Read the model definition and answer for the solid it produces. Units are mm, in the model's axes. A direction names the side the tool comes from. Coordinates: 2 decimals unless noted, no trailing zeros. Write each loop counter-clockwise with the first axis right and the second up, starting at its lowest first coordinate (ties: lowest second). Pieces come first, ordered by that corner, then holes. Notation, with made-up numbers: (31, 17) - (35, 17) arc R34 cw to (35, 55) - close; hole circle Ø4 at (87, 8). An arc over 180 degrees is marked (long way). Return JSON: item names as keys, results as strings.
```python
from build123d import *

# Parameters (mm, degrees)
F0_R     = 24
F0_R_2   = 19
F1_DEPTH = 60
F2_R     = 24
F2_R_2   = 19
F3_DEPTH = 10
F4_R     = 24
F4_R_2   = 19
F5_DEPTH = 10
F6_R     = 9
F7_DEPTH = 25


with BuildPart() as f1:
    # F0 (on Front) → F1 (new body, symmetric)
    with BuildSketch(Plane.XZ):
        with BuildLine():
            Line((83, 13.3241766691), (83, 33.3241766691))
            Line((83, 33.3241766691), (-83, 33.3241766691))
            Line((-83, 33.3241766691), (-83, 13.3241766691))
            Line((-83, 13.3241766691), (-36, 13.3241766691))
            Line((-36, 13.3241766691), (-36, -18.6758233309))
            ThreePointArc((-36, -18.6758233309), (0, -54.6758233309), (36, -18.6758233309))
            Line((36, -18.6758233309), (36, 13.3241766691))
            Line((36, 13.3241766691), (83, 13.3241766691))
        make_face()
        with Locations((0, -18.6758233309)):
            Circle(F0_R, mode=Mode.SUBTRACT)
        with Locations((0, -18.6758233309)):
            Circle(F0_R)
        with Locations((0, -18.6758233309)):
            Circle(F0_R_2, mode=Mode.SUBTRACT)
    extrude(amount=F1_DEPTH, both=True)

    # F2 (on face) → F3 (cut)
    with BuildSketch(Plane.XZ.offset(60)):
        with Locations((0, -18.6758233309)):
            Circle(F2_R)
        with Locations((0, -18.6758233309)):
            Circle(F2_R_2, mode=Mode.SUBTRACT)
    extrude(amount=-F3_DEPTH, mode=Mode.SUBTRACT)

    # F4 (on face) → F5 (cut)
    with BuildSketch(Plane(origin=(0, 60, 0), x_dir=(-1, 0, 0), z_dir=(0, 1, 0))):
        with Locations((0, -18.6758233309)):
            Circle(F4_R)
        with Locations((0, -18.6758233309)):
            Circle(F4_R_2, mode=Mode.SUBTRACT)
    extrude(amount=-F5_DEPTH, mode=Mode.SUBTRACT)

    # F6 (on face) → F7 (cut)
    with BuildSketch(Plane.XY.offset(33.3241766691)):
        with Locations((-59, -32)):
            Circle(F6_R)
        with Locations((-59, 32)):
            Circle(F6_R)
        with Locations((59, -32)):
            Circle(F6_R)
        with Locations((59, 32)):
            Circle(F6_R)
    extrude(amount=-F7_DEPTH, mode=Mode.SUBTRACT)


solid = f1.part
```
(1) Determine the mould class of faces 1 (the face through (63.84, 39.59, 23.46)), 2 (the face through (36, -1, -3)), 3 (the face through (59, -1, 13.324)) for opening direction X: +X half, -X half, draft (parallel to the pull), parting line (faces both ways), or undercut.
Answer:
{"face 1": "undercut", "face 2": "+X half", "face 3": "draft"}
(2) A cutting plane is placed at D-D (z = -10). Determine the outline of the cut face in (x, y), and give its area (3 significant figures).
Answer:
{"outline": "(-36, -60) - (-22.38, -60) - (-22.38, -50) - (-16.9, -50) - (-16.9, 50) - (-22.38, 50) - (-22.38, 60) - (-36, 60) - close; (16.9, -50) - (22.38, -50) - (22.38, -60) - (36, -60) - (36, 60) - (22.38, 60) - (22.38, 50) - (16.9, 50) - close", "area": "4,360 mm²"}
(3) Which of the six approach directions +Z, -Z, +X, -X, +Y, -Y give full straight-line access (tool end or side, diameter ignored) to faces 4 (the face through (-3.12, -55.07, 5.12)), 5 (the face through (3.12, 55.07, 5.12)), 6 (the face through (1, -1, 33.324)), 7 (the face through (-36, -1, -2))?
Answer:
{"face 4": "-Y", "face 5": "+Y", "face 6": "+Z, +X, -X, +Y, -Y", "face 7": "-Z, -X, +Y, -Y"}
(4) Flat-ended cylindrical pins translate along their axes: P1, Ø16, axis at y = -1.5, z = -6.5, coming from the -X side; P2, Ø4, axis at x = 40.5, y = -28.5, coming from the -Z side; P3, Ø2, axis at x = 9, y = -22, coming from the -Z side. Find the tip coordinate at first contact, or state that the pin passes through.
Answer:
{"P1": "x = -36", "P2": "z = 13.32", "P3": "z = -53.78"}
(5) A cutting plane is placed at A-A (y = -32). Determine the outline of the cut face in (x, z).
Answer:
{"outline": "(-83, 13.32) - (-68, 13.32) - (-68, 33.32) - (-83, 33.32) - close; (-50, 13.32) - (-36, 13.32) - (-36, -18.68) arc R36 ccw to (36, -18.68) - (36, 13.32) - (50, 13.32) - (50, 33.32) - (-50, 33.32) - close; (68, 13.32) - (83, 13.32) - (83, 33.32) - (68, 33.32) - close; hole circle Ø38 at (0, -18.68)"}
(6) A cutting plane is placed at C-C (x = 0). Determine the outline of the cut face in (y, z), and give its area (3 significant figures).
Answer:
{"outline": "(-60, -54.68) - (60, -54.68) - (60, -42.68) - (50, -42.68) - (50, -37.68) - (-50, -37.68) - (-50, -42.68) - (-60, -42.68) - close; (-60, 5.32) - (-50, 5.32) - (-50, 0.32) - (50, 0.32) - (50, 5.32) - (60, 5.32) - (60, 33.32) - (-60, 33.32) - close", "area": "5,800 mm²"}
(7) Straight lines are drawn through the part: line 1 (Z direction, x = 0, y = -52.5); line 2 (Y direction, x = -59, z = 28); line 3 (X direction, y = -39, z = 15). For each, find the intervals that lie inside material, in ascending order. Write a range as from..to.
Answer:
{"line 1": "-54.68..-42.68, 5.32..33.32", "line 2": "-60..-41, -23..23, 41..60", "line 3": "-83..-64.66, -53.34..53.34, 64.66..83"}
(8) A cutting plane is placed at B-B (x = -59). Determine the outline of the cut face in (y, z), and give its area (3 significant figures).
Answer:
{"outline": "(-60, 13.32) - (-41, 13.32) - (-41, 33.32) - (-60, 33.32) - close; (-23, 13.32) - (23, 13.32) - (23, 33.32) - (-23, 33.32) - close; (41, 13.32) - (60, 13.32) - (60, 33.32) - (41, 33.32) - close", "area": "1,680 mm²"}
